Here's how the part is built. I have some questions about the finished solid (model axes, mm). A direction names the side the tool comes from. Give positions to 0.01 mm unless a question says otherwise; leave off trailing zeros. Loops run counter-clockwise (first coordinate to the right, second up) from the corner with the lowest first, then second, coordinate; pieces in that order, holes last. Notation, with made-up numbers: (10, 2) - (34, 2) arc R25 cw to (34, 25) - close; hole circle Ø5 at (-31, 13). An arc over 180 degrees is marked (long way). Use a Markdown table: item, result.
from build123d import *

# Parameters (mm, degrees)
F1_R     = 4.7625
F1_R_2   = 15.875
F1_R_3   = 6.096
F1_R_4   = 45.72
F2_DEPTH = 25.4


with BuildPart() as f2:
    # F1 (on face) → F2 (new body)
    with BuildSketch(Plane.XZ):
        Polygon((-47.625, 64.844321), (-87.302212, 53.469552), (-76.2, 0), (-87.297388, -53.469552), (-47.625, -64.844321), (-25.4, -133.35), (25.4, -133.35), (47.625, -64.844321), (87.302212, -53.469552), (76.2, 0), (87.302212, 53.469552), (47.625, 64.844321), (25.4, 133.35), (-25.4, 133.35), align=None)
        with Locations((-73.643908, -45.106811)):
            Circle(F1_R, mode=Mode.SUBTRACT)
        with Locations((-28.75, -49.796461)):
            Circle(F1_R, mode=Mode.SUBTRACT)
        with Locations((0, -96.52)):
            Circle(F1_R_2, mode=Mode.SUBTRACT)
        with Locations((28.75, -49.796461)):
            Circle(F1_R_3, mode=Mode.SUBTRACT)
        with Locations((73.645018, -45.104998)):
            Circle(F1_R, mode=Mode.SUBTRACT)
        with Locations((-57.5, 0)):
            Circle(F1_R_3, mode=Mode.SUBTRACT)
        with Locations((-73.645018, 45.104998)):
            Circle(F1_R, mode=Mode.SUBTRACT)
        with Locations((-28.75, 49.796461)):
            Circle(F1_R, mode=Mode.SUBTRACT)
        Circle(F1_R_4, mode=Mode.SUBTRACT)
        with Locations((28.75, 49.796461)):
            Circle(F1_R_3, mode=Mode.SUBTRACT)
        with Locations((57.5, 0)):
            Circle(F1_R, mode=Mode.SUBTRACT)
        with Locations((73.645018, 45.104998)):
            Circle(F1_R, mode=Mode.SUBTRACT)
        with Locations((0, 96.52)):
            Circle(F1_R_2, mode=Mode.SUBTRACT)
    extrude(amount=F2_DEPTH)


solid = f2.part
(1) We'd pull the mould along X, two halves only. Please class faces 4 (the face through (-2.07, -12.52, 112.26)), 5 (the face through (-36.357, -12.522, 99.577)), 6 (the face through (67.186, -12.522, -59.237)), 7 (the face through (0, -13, 133.35)): pulls with the +X half, pulls with the -X half, needs draft (parallel to the pull), parting line crosses it, or undercut.
A:
| item | result |
|---|---|
| face 4 | undercut |
| face 5 | pulls with the -X half |
| face 6 | pulls with the +X half |
| face 7 | needs draft |
(2) If I drill on line 1 (Z direction, x = 0, y = -20.5) (3 decimals); line 2 (Z direction, x = -4, y = -16.75); line 3 (Z direction, x = -57.5, y = -13), over which ranges is the centre line in solid material (lowest first)?
A:
| item | result |
|---|---|
| line 1 | -133.35 to -112.395, -80.645 to -45.72, 45.72 to 80.645, 112.395 to 133.35 |
| line 2 | -133.35 to -111.88, -81.16 to -45.54, 45.54 to 81.16, 111.88 to 133.35 |
| line 3 | -62.01 to -6.1, 6.1 to 62.01 |
(3) Will these pins go through, and if not, where does the flat tip stop? pin 1 (8 mm diameter, centred on y = -20.5, z = 105, fed in from +X); pin 2 (12 mm diameter, centred on y = -19, z = 16.5, fed in from +X); pin 3 (8 mm diameter, centred on x = 54, y = -15.5, fed in from +Z).
A:
| item | result |
|---|---|
| pin 1 | x = 35.9 |
| pin 2 | x = 80.87 |
| pin 3 | z = 64.16 |
(4) Suppose I cut it at D-D on x = 57.5. Write out the boundary of the cut face in (y, z).
A:
| item | result |
|---|---|
| outline | (-25.4, -62.01) - (0, -62.01) - (0, -4.76) - (-25.4, -4.76) - close; (-25.4, 4.76) - (0, 4.76) - (0, 62.01) - (-25.4, 62.01) - close |
(5) Suppose I cut it at B-B on z = -19.5. Write out the boundary of the cut face in (x, y).
A:
| item | result |
|---|---|
| outline | (-80.25, -25.4) - (-41.35, -25.4) - (-41.35, 0) - (-80.25, 0) - close; (41.35, -25.4) - (80.25, -25.4) - (80.25, 0) - (41.35, 0) - close |
(6) Suppose I cut it at C-C on y = -15.75. Count the separate pieces of the cut face and the enclosed holes in it, plus the area to 3 significant figures.
A:
| item | result |
|---|---|
| separate pieces | 1 |
| enclosed holes | 13 |
| area | 21,600 mm2 |
(7) Suppose I cut it at A-A on x = 0. Write out the boundary of the cut face in (y, z) (3 decimals), plus the area to 3 significant figures.
A:
| item | result |
|---|---|
| outline | (-25.4, -133.35) - (0, -133.35) - (0, -112.395) - (-25.4, -112.395) - close; (-25.4, -80.645) - (0, -80.645) - (0, -45.72) - (-25.4, -45.72) - close; (-25.4, 45.72) - (0, 45.72) - (0, 80.645) - (-25.4, 80.645) - close; (-25.4, 112.395) - (0, 112.395) - (0, 133.35) - (-25.4, 133.35) - close |
| area | 2,840 mm2 |
(8) On a 3-axis mill with a long thin cutter (end or side, diameter ignored), from which of +Z, -Z, +X, -X, +Y, -Y can I reach the whole of each face in a straight line? I mean faces 1 (the face through (-81.67, -12.52, -26.36)), 2 (the face through (81.673, -12.522, 26.36)), 3 (the face through (36.357, -12.522, -99.577)). Say none if no direction works.
A:
| item | result |
|---|---|
| face 1 | -X, +Y, -Y |
| face 2 | +X, +Y, -Y |
| face 3 | -Z, +X, +Y, -Y |
